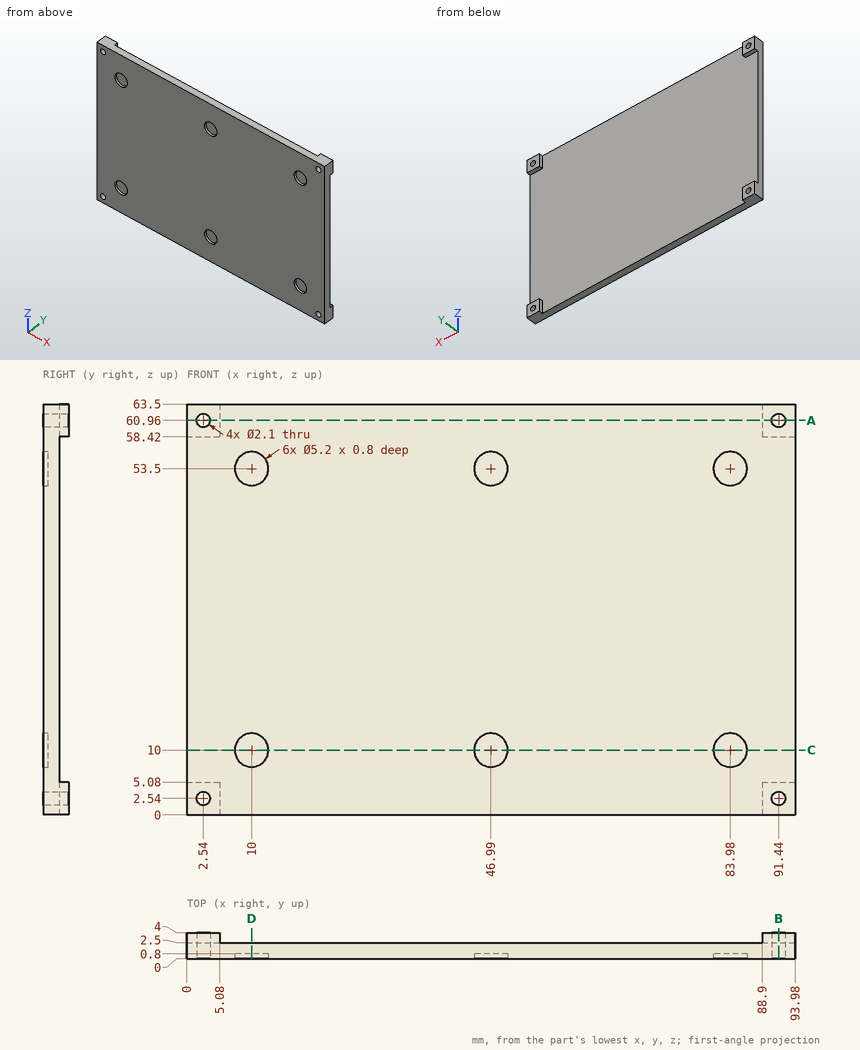
Geometry check sheet. Reference: drawing and pictorial views, mm from the part's lowest x, y, z. Give positions to 0.01 mm unless a question says otherwise; leave off trailing zeros. Order: outer loops, then holes, each group sorted by start corner. A loop starts at its lowest first (then second) coordinate and runs counter-clockwise, first axis right, second up. Notation, with made-up numbers: M -35.75,89.25 L 23.25,89.25 A23 cw 23.25,109.25 Z; hole C 55,-13 d5. An arc over 180 degrees is marked long. Answer in a Markdown table with one row per item. Add a question column.
Q1. Sectioned sample at B-B, the plane x = 91.44. Record the boundary of the cut face in (y, z), and give its area (3 significant figures).
Q2. Sectioned sample at A-A, the plane z = 60.96. Record the boundary of the cut face in (x, y).
Q3. Sectioned sample at C-C, the plane z = 10. Record the boundary of the cut face in (x, y), and give its area (3 significant figures).
Q4. Thickness scan on L1, parallel to X at y = 1.85, z = 60.96; L2, parallel to X at y = 0.5, z = 10; L3, parallel to Z at x = 10.5, y = 0.3. Record the ranges inside material, lowest first.
Q5. Sectioned sample at D-D, the plane x = 10. Record the boundary of the cut face in (y, z), and give its area (3 significant figures).
Q6. Gauge pin test, flat ends, axial feed: pin 1 Ø8.5 at (x, z) = (83.98, 53.5) entering from +Y; pin 2 Ø1.7 at (x, z) = (2.54, 60.96) entering from -Y; pin 3 Ø1.6 at (x, z) = (84, 10) entering from -Y. Record the tip position at first contact, or that the pin passes through.
Verdict:
| question | item | result |
|---|---|---|
| 1 | outline | M 0,0 L 4,0 L 4,1.49 L 0,1.49 Z; M 0,3.59 L 4,3.59 L 4,5.08 L 2.5,5.08 L 2.5,58.42 L 4,58.42 L 4,59.91 L 0,59.91 Z; M 0,62.01 L 4,62.01 L 4,63.5 L 0,63.5 Z |
| 1 | area | 157 mm² |
| 2 | outline | M 0,0 L 1.49,0 L 1.49,4 L 0,4 Z; M 3.59,0 L 90.39,0 L 90.39,4 L 88.9,4 L 88.9,2.5 L 5.08,2.5 L 5.08,4 L 3.59,4 Z; M 92.49,0 L 93.98,0 L 93.98,4 L 92.49,4 Z |
| 3 | outline | M 0,0 L 7.4,0 L 7.4,0.8 L 12.6,0.8 L 12.6,0 L 44.39,0 L 44.39,0.8 L 49.59,0.8 L 49.59,0 L 81.38,0 L 81.38,0.8 L 86.58,0.8 L 86.58,0 L 93.98,0 L 93.98,2.5 L 0,2.5 Z |
| 3 | area | 222 mm² |
| 4 | L1 | 0 to 1.49, 3.59 to 90.39, 92.49 to 93.98 |
| 4 | L2 | 0 to 7.4, 12.6 to 44.39, 49.59 to 81.38, 86.58 to 93.98 |
| 4 | L3 | 0 to 7.45, 12.55 to 50.95, 56.05 to 63.5 |
| 5 | outline | M 0,0 L 2.5,0 L 2.5,63.5 L 0,63.5 L 0,56.1 L 0.8,56.1 L 0.8,50.9 L 0,50.9 L 0,12.6 L 0.8,12.6 L 0.8,7.4 L 0,7.4 Z |
| 5 | area | 150 mm² |
| 6 | pin 1 | y = 2.5 |
| 6 | pin 2 | through |
| 6 | pin 3 | y = 0.8 |
